```python
from build123d import *

# Parameters (mm, degrees)
BOSS_EXTRUDE3_DEPTH = 100
BOSS_EXTRUDE4_REACH = 226.87
SKETCH5_4_R         = 12.5
SKETCH5_4_R_2       = 6
BOSS_EXTRUDE5_DEPTH = 15
SKETCH7_R           = 6
CUT_EXTRUDE1_DEPTH  = 225.869761917
BOSS_EXTRUDE7_DEPTH = 35
CUT_EXTRUDE2_DEPTH  = 8
CUT_EXTRUDE3_DEPTH  = 30


with BuildPart() as part:
    # Sketch4 → Boss-Extrude3 (new body)
    with BuildSketch(Plane.XY):
        Polygon((0, 0), (50, 0), (50, -10), (87.5, -10), (87.5, 0), (112.5, 0), (112.5, -10), (150, -10), (150, 0), (200, 0), (200, 40), (140, 40), (100, 25), (0, 25), align=None)
    extrude(amount=BOSS_EXTRUDE3_DEPTH)

    # Boss-Extrude4: up to this face of the body (flat: up to its plane)
    boss_extrude4_end = Plane(part.part.faces().sort_by_distance((50, 25, 50))[0])
    # Sketch5 → Boss-Extrude4 (add, up to the picked face)
    with BuildSketch(Plane(origin=(0, 54.214936023, 19.732622965), x_dir=(-1, 0, 0), z_dir=(0, 0.9396926207859081, 0.34202014332566943)), mode=Mode.PRIVATE) as boss_extrude4_sk1:
        with BuildLine():
            Line((-15, 85.418758495), (-15, 45.418758495))
            ThreePointArc((-15, 45.418758495), (-40, 20.418758495), (-65, 45.418758495))
            Line((-65, 45.418758495), (-65, 85.418758495))
            Line((-65, 85.418758495), (-15, 85.418758495))
        make_face()
    boss_extrude4_tool1 = split(extrude(boss_extrude4_sk1.sketch, amount=-BOSS_EXTRUDE4_REACH, mode=Mode.PRIVATE), bisect_by=boss_extrude4_end, keep=Keep.BOTH, mode=Mode.PRIVATE)
    add(boss_extrude4_tool1.solids().sort_by(Axis((40, 35.287462, 71.735431), (0, -0.9396926207859081, -0.34202014332566943)))[0])

    # Sketch5<4> → Boss-Extrude5 (add)
    with BuildSketch(Plane(origin=(0, 54.214936023, 19.732622965), x_dir=(-1, 0, 0), z_dir=(0, 0.9396926207859081, 0.34202014332566943))):
        with Locations(Location((-40, 45.418758495, 0), (0, 0, 270))):
            Circle(SKETCH5_4_R)
        with Locations(Location((-40, 45.418758495, 0), (0, 0, 90))):
            Circle(SKETCH5_4_R_2, mode=Mode.SUBTRACT)
    extrude(amount=BOSS_EXTRUDE5_DEPTH)

    # Sketch7 → Cut-Extrude1 (cut, through all)
    with BuildSketch(Plane(origin=(0, 54.214936023, 19.732622965), x_dir=(1, 0, 0), z_dir=(0, 0.9396926207859082, 0.34202014332566943))):
        with Locations(Location((40, -45.418758495, 0), (0, 0, 270))):
            Circle(SKETCH7_R)
    extrude(amount=-CUT_EXTRUDE1_DEPTH, mode=Mode.SUBTRACT)

    # Sketch8 → Boss-Extrude7 (add)
    with BuildSketch(Plane(origin=(14.174682453, -24.551270189, 0), x_dir=(0, 0, -1), z_dir=(0.49999999999999506, -0.8660254037844415, 0))):
        with BuildLine():
            Line((0, 99.102540378), (0, 149.102540378))
            ThreePointArc((0, 149.102540378), (-35, 184.102540378), (-70, 149.102540378))
            Line((-70, 149.102540378), (-70, 99.102540378))
            Line((-70, 99.102540378), (0, 99.102540378))
        make_face()
    extrude(amount=BOSS_EXTRUDE7_DEPTH)

    # Sketch9 → Cut-Extrude2 (cut)
    with BuildSketch(Plane(origin=(14.174682453, -24.551270189, 0), x_dir=(0.8660254037844415, 0.4999999999999951, 0), z_dir=(-0.49999999999999517, 0.8660254037844416, 0))):
        with BuildLine():
            Line((99.102540378, -40), (137.646101141, -40))
            ThreePointArc((137.646101141, -40), (140.241070616, -43.816141653), (144.043854376, -46.430647223))
            Line((144.043854376, -46.430647223), (144.102540378, -70))
            Line((144.102540378, -70), (154.102540378, -70))
            Line((154.102540378, -70), (154.102540378, -46.456439237))
            ThreePointArc((154.102540378, -46.456439237), (157.941375143, -43.838834765), (160.558979616, -40))
            Line((160.558979616, -40), (184.102540378, -40))
            Line((184.102540378, -40), (184.102540378, -30))
            Line((184.102540378, -30), (160.558979616, -30))
            ThreePointArc((160.558979616, -30), (157.941375143, -26.161165235), (154.102540378, -23.543560763))
            Line((154.102540378, -23.543560763), (154.102540378, 0))
            Line((154.102540378, 0), (144.102540378, 0))
            Line((144.102540378, 0), (144.102540378, -23.543560763))
            ThreePointArc((144.102540378, -23.543560763), (140.263705614, -26.161165235), (137.646101141, -30))
            Line((137.646101141, -30), (99.102540378, -30))
            Line((99.102540378, -30), (99.102540378, -40))
        make_face()
    extrude(amount=-CUT_EXTRUDE2_DEPTH, mode=Mode.SUBTRACT)

    # Sketch10 → Cut-Extrude3 (cut)
    with BuildSketch(Plane.XY.offset(100)):
        with BuildLine():
            Line((66.16880238, 26.04463605), (66.16880238, 113.95536395))
            ThreePointArc((66.16880238, 113.95536395), (140, 70), (66.16880238, 26.04463605))
        make_face()
    extrude(amount=-CUT_EXTRUDE3_DEPTH, mode=Mode.SUBTRACT)


solid = part.part
```
Check sheet for the modelled part. Datum: model origin and axes. Units: mm. A direction names the side the tool comes from. Give positions to 0.01 mm unless a question says otherwise; leave off trailing zeros. Order: outer loops, then holes, each group sorted by start corner. A loop starts at its lowest first (then second) coordinate and runs counter-clockwise, first axis right, second up. Notation, with made-up numbers: M 85.25,74.25 L 105.25,74.25 A33 ccw 105.25,105.25 Z; hole C 15,40 d9. An arc over 180 degrees is marked long. Answer in a Markdown table with one row per item. Add a question column.
Q1. Sectioned sample at B-B, the plane z = 9.5. Record the boundary of the cut face in (x, y).
Q2. Thickness scan on L1, parallel to X at y = -1, z = 61; L2, parallel to X at y = 43, z = 66.5; L3, parallel to Z at x = 133, y = 38. Record the ranges inside material, lowest first.
Q3. Sectioned sample at A-A, the plane y = -4. Record the boundary of the cut face in (x, z), and give its area (3 significant figures).
Q4. Gauge pin test, flat ends, axial feed: pin 1 Ø2 at (y, z) = (41.5, 60.5) entering from -X; pin 2 Ø3 at (x, y) = (29, 40) entering from +Z; pin 3 Ø15 at (x, y) = (160, 59.5) entering from +Z; pin 4 Ø22 at (x, y) = (104.5, 40.5) entering from +Z. Record the tip position at first contact, or that the pin passes through.
Q5. Release check for a two-part mould opening along Z. For faces 1 (the cylindrical face through (137.659, 42.188, 26.115)), 2 (the cylindrical face through (39.45, 38.739, 35.836)), 3 (the flat face through (68, -10, 49)) record: released by +Z, released by -Z, zero draft, split by the parting line, or undercut.
Q6. Sectioned sample at D-D, the plane y = 30.5. Count the separate pieces of the cut face and the enclosed holes in it, and give its area (3 significant figures).
Q7. Access from +Z, -Z, +X, -X, +Y, -Y to the whole of each face (thin tool, end or side, straight path). Record for faces 4 (the flat face through (110, 30, 70)), 5 (the flat face through (112.5, -5, 49)), 6 (the flat face through (140.943, 44.084, 11.607)), 7 (the flat face through (34.269, 53.666, 65.097)).
Q8. Sectioned sample at C-C, the plane x = 30. Record the boundary of the cut face in (y, z).
Verdict:
| question | item | result |
|---|---|---|
| 1 | outline | M 0,0 L 50,0 L 50,-10 L 87.5,-10 L 87.5,0 L 112.5,0 L 112.5,-10 L 150,-10 L 150,0 L 200,0 L 200,40 L 176.76,40 L 164.06,61.99 L 147.63,52.5 L 151.63,45.57 L 142.97,40.57 L 138.97,47.5 L 100,25 L 0,25 Z |
| 2 | L1 | 50 to 87.5, 112.5 to 150 |
| 2 | L2 | 27.73 to 34.49, 45.51 to 52.27, 131.18 to 141.56, 147.18 to 164.96 |
| 2 | L3 | 0 to 30, 40 to 70 |
| 3 | outline | M 50,0 L 87.5,0 L 87.5,100 L 50,100 Z; M 112.5,0 L 150,0 L 150,100 L 112.5,100 Z |
| 3 | area | 7,500 mm² |
| 4 | pin 1 | x = 27.62 |
| 4 | pin 2 | z = 71.62 |
| 4 | pin 3 | z = 67.98 |
| 4 | pin 4 | through |
| 5 | face 1 | undercut |
| 5 | face 2 | released by -Z |
| 5 | face 3 | zero draft |
| 6 | separate pieces | 2 |
| 6 | enclosed holes | 1 |
| 6 | area | 10,800 mm² |
| 7 | face 4 | +Z, +Y |
| 7 | face 5 | +Z, -Z, -Y |
| 7 | face 6 | +Z, -Z, +Y |
| 7 | face 7 | +Z, -X, +Y |
| 8 | outline | M 0,0 L 25,0 L 25,33.05 L 46.52,40.88 L 41.25,55.36 L 55.34,60.49 L 50.21,74.59 L 36.12,69.46 L 25,100 L 0,100 Z |
